```python
from build123d import *

# Parameters (mm, degrees)
BOSS_EXTRUDE1_DEPTH = 2
SKETCH2_W           = 18.25
SKETCH2_H           = 1.2
BOSS_EXTRUDE2_DEPTH = 1.2
SKETCH3_W           = 18.25
SKETCH3_H           = 1.2
BOSS_EXTRUDE3_DEPTH = 1.2
FILLET1_R           = 0.1
FILLET2_R           = 0.1
FILLET3_R           = 0.1
FILLET4_R           = 0.1
SKETCH4_R           = 1.41
CUT_EXTRUDE1_DEPTH  = 0.1
BOSS_EXTRUDE4_DEPTH = 4.7
FILLET5_R           = 0.1
SHELL1_START        = 0.710139039
SHELL1_DEPTH        = 77.819860961
SHELL1_START_2      = 1.115016449
SHELL1_2_OUTLINE_W  = 4.49
SHELL1_2_OUTLINE_H  = 0.8
SHELL1_2_DEPTH      = 26.773626454
SHELL1_START_3      = 55.883029025
SHELL1_3_OUTLINE_W  = 4.49
SHELL1_3_OUTLINE_H  = 0.8
SHELL1_3_DEPTH      = 22.646970975
SHELL1_START_4      = 0.8
SHELL1_4_DEPTH      = 4.7
SHELL1_5_DEPTH      = 0.8
SHELL1_START_5      = 0.7
SHELL1_6_OUTLINE_R  = 2.61
SHELL1_6_DEPTH      = 0.1
BOSS_EXTRUDE5_DEPTH = 0.5
SKETCH7_R           = 1.5
BOSS_EXTRUDE6_DEPTH = 3
FILLET6_R           = 0.5
SKETCH8_R           = 0.5
CUT_EXTRUDE2_DEPTH  = 3
SKETCH9_R           = 1.5
BOSS_EXTRUDE7_DEPTH = 3
FILLET7_R           = 0.5
SKETCH10_R          = 0.5
CUT_EXTRUDE3_DEPTH  = 3
FILLET10_R          = 2
FILLET11_R          = 2


with BuildPart() as part:
    # Sketch1 → Boss-Extrude1 (new body)
    with BuildSketch(Plane.XY):
        with BuildLine():
            Line((0, 0), (79.73, 0))
            Line((79.73, 0), (79.73, 7.11))
            ThreePointArc((79.73, 7.11), (76.653638062, 9.862863384), (75.511671928, 13.83))
            Line((75.511671928, 13.83), (58.281671928, 13.83))
            Line((58.281671928, 13.83), (55.245835964, 9.34))
            Line((55.245835964, 9.34), (28.525835964, 9.34))
            Line((28.525835964, 9.34), (25.49, 13.83))
            Line((25.49, 13.83), (11.22, 13.83))
            Line((11.22, 13.83), (1.537833793, 9.231903563))
            Line((1.537833793, 9.231903563), (-0.526918008, 7.167151762))
            Line((-0.526918008, 7.167151762), (0, 0))
        make_face()
    extrude(amount=BOSS_EXTRUDE1_DEPTH)

    # Sketch2 → Boss-Extrude2 (add)
    with BuildSketch(Plane.XZ):
        with Locations((23.625, 1.4)):
            Rectangle(SKETCH2_W, SKETCH2_H)
    extrude(amount=BOSS_EXTRUDE2_DEPTH)

    # Sketch3 → Boss-Extrude3 (add)
    with BuildSketch(Plane.XZ):
        with Locations((57.685, 1.4)):
            Rectangle(SKETCH3_W, SKETCH3_H)
    extrude(amount=BOSS_EXTRUDE3_DEPTH)

    # Fillet1
    fillet1_edges = [part.edges().sort_by_distance(p)[0] for p in [
        (66.81, -1.2, 1.4),
    ]]
    fillet(fillet1_edges, radius=FILLET1_R)

    # Fillet2
    fillet2_edges = [part.edges().sort_by_distance(p)[0] for p in [
        (48.56, -1.2, 1.4),
    ]]
    fillet(fillet2_edges, radius=FILLET2_R)

    # Fillet3
    fillet3_edges = [part.edges().sort_by_distance(p)[0] for p in [
        (32.75, -1.2, 1.4),
    ]]
    fillet(fillet3_edges, radius=FILLET3_R)

    # Fillet4
    fillet4_edges = [part.edges().sort_by_distance(p)[0] for p in [
        (14.5, -1.2, 1.4),
    ]]
    fillet(fillet4_edges, radius=FILLET4_R)

    # Sketch4 → Cut-Extrude1 (cut)
    with BuildSketch(Plane.XY.offset(2)):
        with Locations((24.239473279, 10.02)):
            Circle(SKETCH4_R)
        with Locations((61.560171923, 10.02)):
            Circle(SKETCH4_R)
    extrude(amount=-CUT_EXTRUDE1_DEPTH, mode=Mode.SUBTRACT)

    # Sketch5 → Boss-Extrude4 (add)
    with BuildSketch(Plane.XY.offset(2)):
        with BuildLine():
            Line((75.511671928, 13.83), (72.291671928, 13.83))
            ThreePointArc((72.291671928, 13.83), (73.637392252, 6.559471816), (79.73, 2.37))
            Line((79.73, 2.37), (79.73, 7.11))
            ThreePointArc((79.73, 7.11), (76.653638062, 9.862863384), (75.511671928, 13.83))
        make_face()
    extrude(amount=BOSS_EXTRUDE4_DEPTH)

    # Fillet5
    fillet5_edges = [part.edges().sort_by_distance(p)[0] for p in [
        (76.653638062, 9.862863384, 6.7),
        (73.901671928, 13.83, 6.7),
        (73.637392252, 6.559471816, 6.7),
        (79.73, 4.74, 6.7),
    ]]
    fillet(fillet5_edges, radius=FILLET5_R)

    # Shell1: read off the stored shape, not the designer's step
    # Shell1 outline → Shell1 (cut)
    with BuildSketch(Plane.YZ.offset(SHELL1_START)):
        Polygon((8.14, 0.7), (8.14, 0.8), (1.2, 0.8), (1.2, 0), (8.14, 0), align=None)
    extrude(amount=SHELL1_DEPTH, mode=Mode.SUBTRACT)

    # Shell1 2 outline → Shell1 2 (cut)
    with BuildSketch(Plane.YZ.offset(SHELL1_START_2)):
        with Locations((10.385, 0.4)):
            Rectangle(SHELL1_2_OUTLINE_W, SHELL1_2_OUTLINE_H)
    extrude(amount=SHELL1_2_DEPTH, mode=Mode.SUBTRACT)

    # Shell1 3 outline → Shell1 3 (cut)
    with BuildSketch(Plane.YZ.offset(SHELL1_START_3)):
        with Locations((10.385, 0.4)):
            Rectangle(SHELL1_3_OUTLINE_W, SHELL1_3_OUTLINE_H)
    extrude(amount=SHELL1_3_DEPTH, mode=Mode.SUBTRACT)

    # Shell1 4 outline → Shell1 4 (cut)
    with BuildSketch(Plane.XY.offset(SHELL1_START_4)):
        with BuildLine():
            Line((78.53, 3.991336383), (78.53, 6.394787335))
            ThreePointArc((78.53, 6.394787335), (75.75468216, 9.042947573), (74.395198194, 12.63))
            Line((74.395198194, 12.63), (73.31902509, 12.63))
            ThreePointArc((73.31902509, 12.63), (74.496096812, 7.449025827), (78.53, 3.991336383))
        make_face()
    extrude(amount=SHELL1_4_DEPTH, mode=Mode.SUBTRACT)

    # Shell1 5 outline → Shell1 5 (add)
    with BuildSketch(Plane.XY):
        with BuildLine():
            Line((78.53, 6.394787335), (78.53, 7.835498111))
            ThreePointArc((78.53, 7.835498111), (76.601274587, 9.947529982), (75.608795397, 12.63))
            Line((75.608795397, 12.63), (74.395198194, 12.63))
            ThreePointArc((74.395198194, 12.63), (75.75468216, 9.042947573), (78.53, 6.394787335))
        make_face()
        Polygon((0.710139039, 1.2), (1.115016449, 1.2), (0.710139039, 6.707152534), align=None)
        Polygon((55.883029025, 8.14), (58.918864989, 12.63), (57.47031265, 12.63), (55.883029025, 10.282408245), align=None)
        Polygon((0.710139039, 8.14), (0.710139039, 6.707152534), (2.239820192, 8.236833687), (11.490467063, 12.63), (8.693171864, 12.63), (1.537833793, 9.231903563), (1.115016449, 8.809086219), (1.115016449, 8.14), align=None)
        Polygon((24.852806939, 12.63), (27.888642903, 8.14), (27.888642903, 10.282408245), (26.301359278, 12.63), align=None)
    extrude(amount=SHELL1_5_DEPTH)

    # Shell1 6 outline → Shell1 6 (add)
    with BuildSketch(Plane.XY.offset(SHELL1_START_5)):
        with Locations((61.560171923, 10.02)):
            Circle(SHELL1_6_OUTLINE_R)
        with BuildLine():
            ThreePointArc((24.912484692, 12.541736631), (22.077314607, 8.558093751), (26.830410206, 9.705125674))
            Line((26.830410206, 9.705125674), (24.912484692, 12.541736631))
        make_face()
    extrude(amount=SHELL1_6_DEPTH)

    # Sketch6 → Boss-Extrude5 (add)
    with BuildSketch(Plane(origin=(0, 0, 0.8), x_dir=(-1, 0, 0), z_dir=(0, 0, -1))):
        Polygon((-74.121905242, 8.14), (-2.142986505, 8.14), (-0.942986505, 6.94), (-74.828664694, 6.94), align=None)
    extrude(amount=BOSS_EXTRUDE5_DEPTH)

    # Sketch7 → Boss-Extrude6 (add)
    with BuildSketch(Plane(origin=(0, 0, 0.7), x_dir=(-1, 0, 0), z_dir=(0, 0, -1))):
        with Locations(Location((-61.560171923, 10.02, 0), (0, 0, 180))):
            Circle(SKETCH7_R)
    extrude(amount=BOSS_EXTRUDE6_DEPTH)

    # Fillet6
    fillet6_edges = [part.edges().sort_by_distance(p)[0] for p in [
        (60.060171923, 10.02, -2.3),
    ]]
    fillet(fillet6_edges, radius=FILLET6_R)

    # Sketch8 → Cut-Extrude2 (cut)
    with BuildSketch(Plane(origin=(0, 0, -2.3), x_dir=(-1, 0, 0), z_dir=(0, 0, -1))):
        with Locations((-61.560171923, 10.02)):
            Circle(SKETCH8_R)
    extrude(amount=-CUT_EXTRUDE2_DEPTH, mode=Mode.SUBTRACT)

    # Sketch9 → Boss-Extrude7 (add)
    with BuildSketch(Plane(origin=(0, 0, 0.7), x_dir=(-1, 0, 0), z_dir=(0, 0, -1))):
        with Locations(Location((-24.239473279, 10.02, 0), (0, 0, 180))):
            Circle(SKETCH9_R)
    extrude(amount=BOSS_EXTRUDE7_DEPTH)

    # Fillet7
    fillet7_edges = [part.edges().sort_by_distance(p)[0] for p in [
        (22.739473279, 10.02, -2.3),
    ]]
    fillet(fillet7_edges, radius=FILLET7_R)

    # Sketch10 → Cut-Extrude3 (cut)
    with BuildSketch(Plane(origin=(0, 0, -2.3), x_dir=(-1, 0, 0), z_dir=(0, 0, -1))):
        with Locations((-24.239473279, 10.02)):
            Circle(SKETCH10_R)
    extrude(amount=-CUT_EXTRUDE3_DEPTH, mode=Mode.SUBTRACT)

    # Fillet10
    # the kernel refuses this fillet: 2 mm, written as the material it takes off along each edge
    with BuildSketch(Plane(origin=(81.740835966, 11.819164038, 0.8), x_dir=(-0.7731681215232679, 0.634201116255862, 0), z_dir=(0.634201116255862, 0.7731681215232679, 0))) as fillet10_piece_1_section:
        with BuildLine():
            CenterArc((8.460753713 + FILLET10_R, FILLET10_R), FILLET10_R, 180, 90)
            Line((8.460753713, FILLET10_R), (8.460753713, 0))
            Line((8.460753713, 0), (8.460753713 + FILLET10_R, 0))
        make_face()
    fillet10_piece_1 = revolve(axis=Axis((81.740835966, 11.819164038, 0.8), (0, 0, 1)), revolution_arc=98.997926529, mode=Mode.PRIVATE)
    fillet10_piece_1 = split(fillet10_piece_1, bisect_by=Plane(origin=(81.740835966, 12.63, 0.8), z_dir=(0, -1, 0)), keep=Keep.TOP, mode=Mode.PRIVATE)
    fillet10_piece_1 = split(fillet10_piece_1, bisect_by=Plane(origin=(81.740835966, 8.14, 0.8), z_dir=(0, 1, 0)), keep=Keep.TOP, mode=Mode.PRIVATE)
    add(fillet10_piece_1, mode=Mode.SUBTRACT)

    # Fillet11
    # the kernel refuses this fillet: 2 mm, written as the material it takes off along each edge
    with BuildSketch(Plane(origin=(81.740835966, 11.819164038, 0.8), x_dir=(-0.9997199584304023, -0.023664418774073097, 0), z_dir=(-0.023664418774073097, 0.9997199584304023, 0))) as fillet11_piece_1_section:
        with BuildLine():
            CenterArc((8.460753713 + FILLET11_R, FILLET11_R), FILLET11_R, 180, 90)
            Line((8.460753713, FILLET11_R), (8.460753713, 0))
            Line((8.460753713, 0), (8.460753713 + FILLET11_R, 0))
        make_face()
    fillet11_piece_1 = revolve(axis=Axis((81.740835966, 11.819164038, 0.8), (0, 0, 1)), revolution_arc=100.202942333, mode=Mode.PRIVATE)
    fillet11_piece_1 = split(fillet11_piece_1, bisect_by=Plane(origin=(78.53, 11.819164038, 0.8), z_dir=(-1, 0, 0)), keep=Keep.TOP, mode=Mode.PRIVATE)
    fillet11_piece_1 = split(fillet11_piece_1, bisect_by=Plane(origin=(81.740835966, 6.94, 0.8), z_dir=(0, -1, 0)), keep=Keep.TOP, mode=Mode.PRIVATE)
    add(fillet11_piece_1, mode=Mode.SUBTRACT)


solid = part.part
```
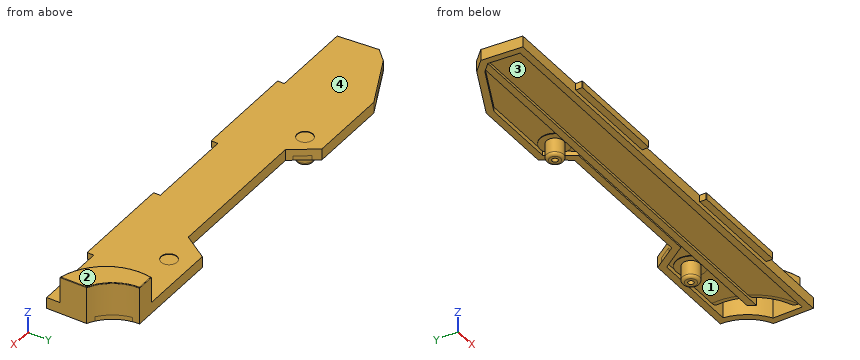
The listing builds one solid part. Answer for the finished solid, in the listing's coordinates (mm). Face numbers are marked on the shaded views. A direction names the side the tool comes from. Round coordinates to 2 decimals unless told otherwise and drop trailing zeros. Order: outer loops, then holes, each group sorted by start corner. A loop starts at its lowest first (then second) coordinate and runs counter-clockwise, first axis right, second up. Notation, with made-up numbers: (14, 62) -> (55, 62) arc R25 cw to (55, 79) -> close; hole circle Ø2 at (-26.75, -2). An arc over 180 degrees is marked (long way). Answer as CSV lines item,"result". Start each with the question number.
(1) The part is cut by section B-B (z = 4.5). Determine the outline of the cut face in (x, y).
(2) A tool of negligible diameter and unlimited length cuts with its end or side. For the marked faces 1 and 2, from which of +Z, -Z, +X, -X, +Y, -Y can it reach the whole face along a straight path? Write none if from no direction.
(3) For a pull along Y with two mould halves and no side action, classify the marked faces 3 and 4 as +Y half, -Y half, draft (parallel to the pull), parting line (faces both ways), or undercut.
(4) The part is cut by section C-C (x = 37). Determine the outline of the cut face in (y, z).
(5) The part is cut by section A-A (x = 70.5). Determine the outline of the cut face in (y, z).
(6) Flat-ended cylindrical pins translate along their axes: pin 1 Ø3 at (y, z) = (5, -0.5) entering from -X; pin 2 Ø1 at (x, y) = (60, -1) entering from -Z; pin 3 Ø0.8 at (x, y) = (61.5, 9.5) entering from +Z. Find the tip coordinate at first contact, or state that the pin passes through.
(7) Find the intervals of material crossed by probe 1 along Y at (x, z) = (17, 0.75); probe 2 along X at (y, z) = (10.5, 1.5); probe 3 along Z at (x, y) = (24, 13.25), in increasing order. Write a range as from..to.
Evaluation:
1,outline,"(72.29, 13.83) arc R9.66 ccw to (79.73, 2.37) -> (79.73, 7.11) arc R7.46 cw to (75.51, 13.83) -> close; hole (73.32, 12.63) arc R8.46 ccw to (78.53, 3.99) -> (78.53, 6.39) arc R8.66 cw to (74.4, 12.63) -> close"
2,face 1,"-Z"
2,face 2,"+Z, +X, -X, +Y, -Y"
3,face 3,"undercut"
3,face 4,"draft"
4,outline,"(0, 0) -> (1.2, 0) -> (1.2, 0.8) -> (6.94, 0.8) -> (6.94, 0.3) -> (8.14, 0.3) -> (8.14, 0) -> (9.34, 0) -> (9.34, 2) -> (0, 2) -> close"
5,outline,"(0, 0) -> (1.2, 0) -> (1.2, 0.8) -> (6.94, 0.8) -> (6.94, 0.3) -> (8.14, 0.3) -> (8.14, 0.8) -> (12.63, 0.8) -> (12.63, 0) -> (13.83, 0) -> (13.83, 2) -> (0, 2) -> close"
6,pin 1,"x = -0.47"
6,pin 2,"z = 0.8"
6,pin 3,"z = 1.9"
7,probe 1,"0..1.2, 6.94..8.14, 12.63..13.83"
7,probe 2,"4.21..27.74, 56.03..72.9, 74.98..76.3"
7,probe 3,"0..2"
